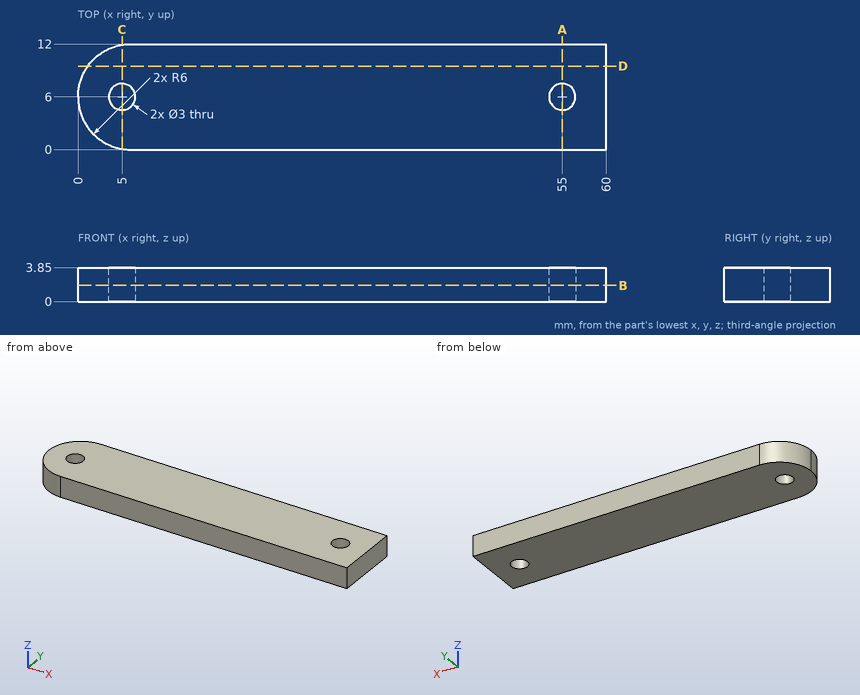
Answer from the drawing. Dimensions are ordinates in mm from the lowest x, y and z of the part. Coordinates: 2 decimals unless noted, no trailing zeros. Order: outer loops, then holes, each group sorted by start corner. A loop starts at its lowest first (then second) coordinate and runs counter-clockwise, first axis right, second up. Notation, with made-up numbers: (80, -24) - (92, -24) arc R21 cw to (92, 12) - close; hole circle Ø10 at (13.5, 64). An arc over 180 degrees is marked (long way). Put each result on its own line as item: value. Start each with the question number.
1) Find section A-A (x = 55). Give the vertices of the cut face in (y, z).
2) Find section C-C (x = 5). Give the vertices of the cut face in (y, z).
3) Find section B-B (z = 1.85). State how many separate pieces and enclosed holes the cut face has, plus the area to 3 significant figures.
4) Find the intervals of material crossed by line 1 (Y direction, x = 55, z = 1.45); line 2 (Y direction, x = 5, z = 1.1); line 3 (X direction, y = 1, z = 2.9), in increasing order. Write a range as from..to.
5) Find section D-D (y = 9.5). Give the vertices of the cut face in (x, z).
Results list:
1. outline: (0, 0) - (4.5, 0) - (4.5, 3.85) - (0, 3.85) - close; (7.5, 0) - (12, 0) - (12, 3.85) - (7.5, 3.85) - close
2. outline: (0.08, 0) - (4.5, 0) - (4.5, 3.85) - (0.08, 3.85) - close; (7.5, 0) - (11.92, 0) - (11.92, 3.85) - (7.5, 3.85) - close
3. separate pieces: 1
3. enclosed holes: 2
3. area: 690 mm^2
4. line 1: y = 0..4.5, 7.5..12
4. line 2: y = 0.08..4.5, 7.5..11.92
4. line 3: x = 2.68..60
5. outline: (1.13, 0) - (60, 0) - (60, 3.85) - (1.13, 3.85) - close
